The listing builds one solid part. Answer for the finished solid, in the listing's coordinates (mm). A direction names the side the tool comes from. Give positions to 0.01 mm unless a question says otherwise; leave off trailing zeros. Write each loop counter-clockwise with the first axis right and the second up, starting at its lowest first coordinate (ties: lowest second). Pieces come first, ordered by that corner, then holes.
```python
from build123d import *

# Parameters (mm, degrees)
SKETCH1_W           = 147
SKETCH1_H           = 105
BOSS_EXTRUDE4_DEPTH = 40
BOSS_EXTRUDE5_DEPTH = 12.7
CUT_EXTRUDE3_DEPTH  = 10.16
BOSS_EXTRUDE6_DEPTH = 12.7
CUT_EXTRUDE4_DEPTH  = 10.16


with BuildPart() as part:
    # Sketch1 → Boss-Extrude4 (new body)
    with BuildSketch(Plane.XY):
        Rectangle(SKETCH1_W, SKETCH1_H)
    extrude(amount=BOSS_EXTRUDE4_DEPTH)

    # Sketch6 → Boss-Extrude5 (add)
    with BuildSketch(Plane.ZY.offset(73.5)):
        with BuildLine():
            Line((9.360303109, 3.859497892), (9.360303109, 37.656182133))
            ThreePointArc((9.360303109, 37.656182133), (19.165513969, 47.461392993), (28.970724829, 37.656182133))
            Line((28.970724829, 37.656182133), (28.970724829, 3.859497892))
            ThreePointArc((28.970724829, 3.859497892), (19.165513969, -5.945712968), (9.360303109, 3.859497892))
        make_face()
    extrude(amount=BOSS_EXTRUDE5_DEPTH)

    # Sketch7 → Cut-Extrude3 (cut)
    with BuildSketch(Plane.ZY.offset(86.2)):
        with BuildLine():
            Line((12.154400228, 3.770764543), (11.749992656, 37.567448784))
            ThreePointArc((11.749992656, 37.567448784), (19.076780621, 45.071703446), (26.581035283, 37.744915482))
            Line((26.581035283, 37.744915482), (26.985442854, 3.94823124))
            ThreePointArc((26.985442854, 3.94823124), (19.65865489, -3.556023421), (12.154400228, 3.770764543))
        make_face()
    extrude(amount=-CUT_EXTRUDE3_DEPTH, mode=Mode.SUBTRACT)

    # Sketch8 → Boss-Extrude6 (add)
    with BuildSketch(Plane.ZY.offset(73.5)):
        with BuildLine():
            Line((10.403410648, -38.907911179), (10.403410648, -20.549218505))
            ThreePointArc((10.403410648, -20.549218505), (19.582756985, -11.369872168), (28.762103322, -20.549218505))
            Line((28.762103322, -20.549218505), (28.762103322, -38.907911179))
            ThreePointArc((28.762103322, -38.907911179), (19.582756985, -48.087257516), (10.403410648, -38.907911179))
        make_face()
    extrude(amount=BOSS_EXTRUDE6_DEPTH)

    # Sketch9 → Cut-Extrude4 (cut)
    with BuildSketch(Plane.ZY.offset(86.2)):
        with BuildLine():
            Line((12.388273633, -38.928322069), (12.336561358, -20.569629395))
            ThreePointArc((12.336561358, -20.569629395), (19.562346094, -13.303022878), (26.828952612, -20.528807614))
            Line((26.828952612, -20.528807614), (26.880664887, -38.887500288))
            ThreePointArc((26.880664887, -38.887500288), (19.654880151, -46.154106806), (12.388273633, -38.928322069))
        make_face()
    extrude(amount=-CUT_EXTRUDE4_DEPTH, mode=Mode.SUBTRACT)


solid = part.part
```
Item 1: A cutting plane is placed at D-D, the plane z = 4.5. Give the vertices of the cut face in (x, y).
Conclusion:
outline: (-73.5, -52.5) - (73.5, -52.5) - (73.5, 52.5) - (-73.5, 52.5) - close
Item 2: A cutting plane is placed at B-B, the plane z = 21.5. Give the vertices of the cut face in (x, y), plus the area to 3 significant figures.
Conclusion:
outline: (-86.2, -47.88) - (-73.5, -47.88) - (-73.5, -52.5) - (73.5, -52.5) - (73.5, 52.5) - (-73.5, 52.5) - (-73.5, 47.18) - (-86.2, 47.18) - (-86.2, 44.7) - (-76.04, 44.7) - (-76.04, -3.3) - (-86.2, -3.3) - (-86.2, -5.66) - (-73.5, -5.66) - (-73.5, -11.57) - (-86.2, -11.57) - (-86.2, -13.56) - (-76.04, -13.56) - (-76.04, -45.91) - (-86.2, -45.91) - close
area: 15,800 mm2
Item 3: A cutting plane is placed at A-A, the plane y = -41. Give the vertices of the cut face in (x, z) (3 decimals).
Conclusion:
outline: (-86.2, 10.645) - (-73.5, 10.645) - (-73.5, 0) - (73.5, 0) - (73.5, 40) - (-73.5, 40) - (-73.5, 28.521) - (-86.2, 28.521) - (-86.2, 26.572) - (-76.04, 26.572) - (-76.04, 12.697) - (-86.2, 12.697) - close
Item 4: Determine the mould class of faces 4 (the face through (-76.04, 21, 19)), 5 (the face through (-1, 1, 0)), 6 (the face through (-1, 52.5, 20)), 7 (the face through (-81.191, -46.152, 19.814)) for opening direction Y: pulls with the +Y half, pulls with the -Y half, needs draft (parallel to the pull), parting line crosses it, or undercut.
Conclusion:
face 4: undercut
face 5: needs draft
face 6: pulls with the +Y half
face 7: undercut
Item 5: Each of these flat-tipped pins is pushed along its axis until it touches: P1, Ø6.5, axis at x = -79, y = 17, coming from the -Z side; P2, Ø4, axis at x = -82, y = 24.5, coming from the +Z side; P3, Ø7.5, axis at y = -29, z = 22.5, coming from the -X side. Where does it stop, or does it pass through?
Conclusion:
P1: stops at z = 9.36
P2: stops at z = 28.97
P3: stops at x = -76.04
Item 6: Consider probe 1 along X at (y, z) = (-13, 29); probe 2 along X at (y, z) = (-27.5, 17); probe 3 along Z at (x, y) = (-77, -2). Determine where each line is inside the solid, lowest interval first.
Conclusion:
probe 1: x = -73.5 to 73.5
probe 2: x = -76.04 to 73.5
probe 3: z = 11.3 to 15.02, 24.12 to 27.03
Item 7: Which of the six approach directions +Z, -Z, +X, -X, +Y, -Y give full straight-line access (tool end or side, diameter ignored) to faces 1 (the face through (-80, 21, 9.36)), 2 (the face through (-80, 21, 28.971)), 3 (the face through (-79.761, -48.085, 19.785))?
Conclusion:
face 1: -Z, -X, +Y, -Y
face 2: +Z, -X, +Y, -Y
face 3: -X, -Y
Item 8: A cutting plane is placed at C-C, the plane y = 13.5. Give the vertices of the cut face in (x, z), plus the area to 3 significant figures.
Conclusion:
outline: (-86.2, 9.36) - (-73.5, 9.36) - (-73.5, 0) - (73.5, 0) - (73.5, 40) - (-73.5, 40) - (-73.5, 28.97) - (-86.2, 28.97) - (-86.2, 26.87) - (-76.04, 26.87) - (-76.04, 12.04) - (-86.2, 12.04) - close
area: 5,980 mm2
